Model file for the job. Use its own axes, mm. Coordinates: 2 decimals unless noted, no trailing zeros. Order: outer loops, then holes, each group sorted by start corner. A loop starts at its lowest first (then second) coordinate and runs counter-clockwise, first axis right, second up. Notation, with made-up numbers: (20.25, -5) -> (29.25, -5) arc R17 cw to (29.25, 27) -> close; hole circle Ø4 at (44, 12.25). An arc over 180 degrees is marked (long way). Return JSON: item names as keys, results as strings. Group by question number.
1) Cut at D-D (x = 12.75). Write the cut outline in (y, z), and give its area (3 significant figures).
2) Cut at A-A (y = 80). Write the cut outline in (x, z), and give its area (3 significant figures).
3) Probe line 1 (X direction, y = 44, z = 1.05); line 2 (Y direction, x = 5, z = 1.75); line 3 (Y direction, x = 12, z = 0.2). List the from-to ranges inside material, lowest first.
4) Flat gauge pins, fed straight in: pin 1 (7 mm diameter, centred on x = 0, y = 50, fed in from +Z); pin 2 (5.5 mm diameter, centred on x = 0, y = 110, fed in from +Z); pin 3 (0.6 mm diameter, centred on y = 83, z = 1, fed in from -X); pin 4 (0.8 mm diameter, centred on x = 14.5, z = 1, fed in from +Y). Where does each tip first touch, or does it go through?
5) Pull direction Y, two halves, no side cores. Call faces 1 (the flat face through (0, 57, 2)), 2 (the cylindrical face through (-2.4, 108.2, 1)), 3 (the cylindrical face through (9, 22.1, 1)): +Y half, -Y half, draft (parallel to the pull), parting line (faces both ways), or undercut.
6) Cut at C-C (y = 100). Write the cut outline in (x, z).
7) Cut at B-B (z = 0.95). Write the cut outline in (x, y), and give its area (3 significant figures).
from build123d import *

# Parameters (mm, degrees)
PAD_DEPTH   = 2
SKETCH001_R = 3
HOLE_DEPTH  = 25


with BuildPart() as part:
    # Sketch → Pad (new body)
    with BuildSketch(Plane.XY):
        with BuildLine():
            Line((0, 0), (15, 0))
            Line((15, 0), (15, 20))
            Line((14, 20), (15, 20))
            ThreePointArc((7, 26.999996), (9.050254, 22.050251), (14, 20))
            Line((7, 28.739996), (7, 26.999996))
            Line((7, 132.311423), (7, 28.739996))
            ThreePointArc((7, 132.311422), (5.133926, 139.557111), (0, 145))
            Line((0, 145), (0, 0))
        make_face()
    pad = extrude(amount=PAD_DEPTH)

    # Mirrored: Pad across Sketch V_Axis
    add(pad.mirror(Plane(origin=(0, 0, 0), x_dir=(0, 0, 1), z_dir=(1, 0, 0))))

    # Sketch001 (on Face5 of Mirrored) → Hole (cut)
    with BuildSketch(Plane.XY.offset(2)):
        with Locations((0, 35)):
            Circle(SKETCH001_R)
        with Locations((0, 50)):
            Circle(SKETCH001_R)
        with Locations((0, 65)):
            Circle(SKETCH001_R)
        with Locations((0, 80)):
            Circle(SKETCH001_R)
        with Locations((0, 95)):
            Circle(SKETCH001_R)
        with Locations((0, 110)):
            Circle(SKETCH001_R)
        with Locations((0, 125)):
            Circle(SKETCH001_R)
    extrude(amount=-HOLE_DEPTH, mode=Mode.SUBTRACT)


solid = part.part
Answers below:
{
 "1": {"outline": "(0, 0) -> (20.11, 0) -> (20.11, 2) -> (0, 2) -> close", "area": "40.2 mm^2"},
 "2": {"outline": "(-7, 0) -> (-3, 0) -> (-3, 2) -> (-7, 2) -> close; (3, 0) -> (7, 0) -> (7, 2) -> (3, 2) -> close", "area": "16.0 mm^2"},
 "3": {"line 1": "x = -7 to 7", "line 2": "y = 0 to 139.79", "line 3": "y = 0 to 20.29"},
 "4": {"pin 1": "stops at z = 2", "pin 2": "passes through", "pin 3": "stops at x = -7", "pin 4": "stops at y = 20"},
 "5": {"face 1": "draft", "face 2": "undercut", "face 3": "+Y half"},
 "6": {"outline": "(-7, 0) -> (7, 0) -> (7, 2) -> (-7, 2) -> close"},
 "7": {"outline": "(-15, 0) -> (15, 0) -> (15, 20) -> (14, 20) arc R7 cw to (7, 27) -> (7, 132.31) arc R15 ccw to (0, 145) arc R15 ccw to (-7, 132.31) -> (-7, 27) arc R7 cw to (-14, 20) -> (-15, 20) -> close; hole circle Ø6 at (0, 35); hole circle Ø6 at (0, 50); hole circle Ø6 at (0, 65); hole circle Ø6 at (0, 80); hole circle Ø6 at (0, 95); hole circle Ø6 at (0, 110); hole circle Ø6 at (0, 125)", "area": "2,120 mm^2"}
}
